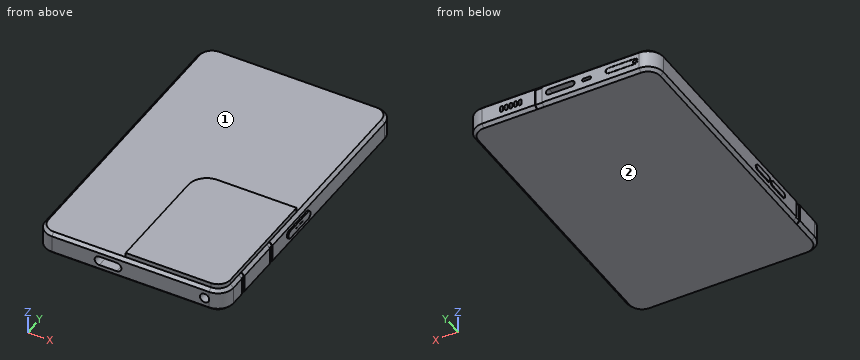
```python
from build123d import *

# Parameters (mm, degrees)
EXTRUDE_1_DEPTH        = 15
CHAMFER_7_SIZE         = 2
CHAMFER_8_SIZE         = 2
CUT_EXTRUDE_1_DEPTH    = 6
PATTERN_LINEAR_1_COUNT = 5
PATTERN_LINEAR_1_PITCH = 3
CUT_EXTRUDE_2_DEPTH    = 10
CUT_EXTRUDE_3_DEPTH    = 40
CUT_EXTRUDE_5_DEPTH    = 20
EXTRUDE_2_DEPTH        = 20
SKETCH_9_R             = 1.114563032
CUT_EXTRUDE_6_DEPTH    = 20
SKETCH_10_R            = 2.990185925
CUT_EXTRUDE_8_DEPTH    = 20
SKETCH_12_W            = 4.560479379
SKETCH_12_H            = 11
CUT_EXTRUDE_9_DEPTH    = 0.5
SKETCH_13_W            = 4.560479379
SKETCH_13_H            = 2.828427125
CUT_EXTRUDE_10_DEPTH   = 0.5
SKETCH_14_W            = 4.560479379
SKETCH_14_H            = 2.828427125
CUT_EXTRUDE_11_DEPTH   = 0.5
EXTRUDE_3_DEPTH        = 1
EXTRUDE_4_DEPTH        = 0.1
SKETCH_17_W            = 11
SKETCH_17_H            = 3
CUT_EXTRUDE_12_DEPTH   = 0.5
SKETCH_18_W            = 2.828427124
SKETCH_18_H            = 3
CUT_EXTRUDE_13_DEPTH   = 0.5
SKETCH_19_W            = 2.828427124
SKETCH_19_H            = 3
CUT_EXTRUDE_14_DEPTH   = 0.5
EXTRUDE_5_DEPTH        = 0.5
SKETCH_26_W            = 11
SKETCH_26_H            = 4
CUT_EXTRUDE_15_DEPTH   = 0.5
SKETCH_27_W            = 2.828427124
SKETCH_27_H            = 4
CUT_EXTRUDE_16_DEPTH   = 0.5
SKETCH_28_W            = 2.828427124
SKETCH_28_H            = 4
CUT_EXTRUDE_17_DEPTH   = 0.5
EXTRUDE_6_DEPTH        = 3


with BuildPart() as part:
    # 草图1 → 凸台-拉伸1 (new body)
    with BuildSketch(Plane.XY):
        with BuildLine():
            Line((-50.87521941, 95.847945747), (50.87521941, 95.847945747))
            ThreePointArc((50.87521941, 95.847945747), (57.946287222, 92.919013559), (60.87521941, 85.847945747))
            Line((60.87521941, 85.847945747), (60.87521941, -85.847945747))
            ThreePointArc((60.87521941, -85.847945747), (57.946287222, -92.919013559), (50.87521941, -95.847945747))
            Line((50.87521941, -95.847945747), (-50.87521941, -95.847945747))
            ThreePointArc((-50.87521941, -95.847945747), (-57.946287222, -92.919013559), (-60.87521941, -85.847945747))
            Line((-60.87521941, -85.847945747), (-60.87521941, 85.847945747))
            ThreePointArc((-60.87521941, 85.847945747), (-57.946287222, 92.919013559), (-50.87521941, 95.847945747))
        make_face()
    extrude(amount=EXTRUDE_1_DEPTH)

    # 倒角7
    chamfer_7_edges = [part.edges().sort_by_distance(p)[0] for p in [
        (0, 95.847945747, 0),
        (57.946287222, 92.919013559, 0),
        (60.87521941, 0, 0),
        (57.946287222, -92.919013559, 0),
        (0, -95.847945747, 0),
        (-57.946287222, -92.919013559, 0),
        (-60.87521941, 0, 0),
        (-57.946287222, 92.919013559, 0),
    ]]
    chamfer(chamfer_7_edges, length=CHAMFER_7_SIZE)

    # 倒角8
    chamfer_8_edges = [part.edges().sort_by_distance(p)[0] for p in [
        (57.946287222, 92.919013559, 15),
        (0, 95.847945747, 15),
        (-57.946287222, 92.919013559, 15),
        (-60.87521941, 0, 15),
        (-57.946287222, -92.919013559, 15),
        (0, -95.847945747, 15),
        (57.946287222, -92.919013559, 15),
        (60.87521941, 0, 15),
    ]]
    chamfer(chamfer_8_edges, length=CHAMFER_8_SIZE)

    # 草图4 → 切除-拉伸1 (cut)
    with BuildSketch(Plane(origin=(0, 95.847945747, 0), x_dir=(1, 0, 0), z_dir=(0, 1, 0))):
        with BuildLine():
            Line((25.184922723, -6.52592521), (25.184922723, -8.52592521))
            ThreePointArc((25.184922723, -8.52592521), (26.184922723, -9.52592521), (27.184922723, -8.52592521))
            Line((27.184922723, -8.52592521), (27.184922723, -6.52592521))
            ThreePointArc((27.184922723, -6.52592521), (26.184922723, -5.52592521), (25.184922723, -6.52592521))
        make_face()
    cut_extrude_1 = extrude(amount=-CUT_EXTRUDE_1_DEPTH, mode=Mode.SUBTRACT)

    # 阵列(线性)1: 切除-拉伸1 ×5
    with Locations(*[(i * PATTERN_LINEAR_1_PITCH, 0, 0) for i in range(1, PATTERN_LINEAR_1_COUNT)]):
        add(cut_extrude_1, mode=Mode.SUBTRACT)

    # 草图5 → 切除-拉伸2 (cut)
    with BuildSketch(Plane(origin=(0, 95.847945747, 0), x_dir=(1, 0, 0), z_dir=(0, 1, 0))):
        with BuildLine():
            Line((-18.674903906, -6.52592521), (-14.956626917, -6.52592521))
            ThreePointArc((-14.956626917, -6.52592521), (-13.956626917, -7.52592521), (-14.956626917, -8.52592521))
            Line((-14.956626917, -8.52592521), (-18.674903906, -8.52592521))
            ThreePointArc((-18.674903906, -8.52592521), (-19.674903906, -7.52592521), (-18.674903906, -6.52592521))
        make_face()
    extrude(amount=-CUT_EXTRUDE_2_DEPTH, mode=Mode.SUBTRACT)

    # 草图6 → 切除-拉伸3 (cut)
    with BuildSketch(Plane(origin=(0, 95.847945747, 0), x_dir=(1, 0, 0), z_dir=(0, 1, 0))):
        with BuildLine():
            Line((-7.094079035, -5.954899544), (7.600798966, -5.954899544))
            ThreePointArc((7.600798966, -5.954899544), (9.543225368, -7.897325947), (7.600798966, -9.839752349))
            Line((7.600798966, -9.839752349), (-7.094079035, -9.839752349))
            ThreePointArc((-7.094079035, -9.839752349), (-9.036505437, -7.897325947), (-7.094079035, -5.954899544))
        make_face()
    extrude(amount=-CUT_EXTRUDE_3_DEPTH, mode=Mode.SUBTRACT)

    # 草图7 → 切除-拉伸5 (cut)
    with BuildSketch(Plane(origin=(0, 95.847945747, 0), x_dir=(1, 0, 0), z_dir=(0, 1, 0))):
        with BuildLine():
            Line((-47.943352298, -5.954899544), (-31.050839612, -5.954899544))
            ThreePointArc((-31.050839612, -5.954899544), (-29.108413209, -7.897325947), (-31.050839612, -9.839752349))
            Line((-31.050839612, -9.839752349), (-47.943352298, -9.839752349))
            ThreePointArc((-47.943352298, -9.839752349), (-49.885778701, -7.897325947), (-47.943352298, -5.954899544))
        make_face()
    extrude(amount=-CUT_EXTRUDE_5_DEPTH, mode=Mode.SUBTRACT)

    # 草图8 → 凸台-拉伸2 (add)
    with BuildSketch(Plane(origin=(0, 75.847945747, 0), x_dir=(1, 0, 0), z_dir=(0, 1, 0))):
        with BuildLine():
            Line((-47.943352298, -6.108012441), (-31.050839612, -6.108012441))
            ThreePointArc((-31.050839612, -6.108012441), (-29.259969658, -7.898882395), (-31.050839612, -9.689752349))
            Line((-31.050839612, -9.689752349), (-47.943352298, -9.689752349))
            ThreePointArc((-47.943352298, -9.689752349), (-49.734222253, -7.898882395), (-47.943352298, -6.108012441))
        make_face()
    extrude(amount=EXTRUDE_2_DEPTH)

    # 草图9 → 切除-拉伸6 (cut)
    with BuildSketch(Plane(origin=(0, 95.847945747, 0), x_dir=(1, 0, 0), z_dir=(0, 1, 0))):
        with Locations(Location((-47.943352298, -7.898882395, 0), (0, 0, 270))):
            Circle(SKETCH_9_R)
    extrude(amount=-CUT_EXTRUDE_6_DEPTH, mode=Mode.SUBTRACT)

    # 草图10 → 切除-拉伸8 (cut)
    with BuildSketch(Plane.XZ.offset(95.847945747)):
        with Locations(Location((47.885033485, 7.5, 0), (0, 0, 270))):
            Circle(SKETCH_10_R)
        with BuildLine():
            Line((-8.945418448, 10.490185925), (-20.268797242, 10.490185925))
            ThreePointArc((-20.268797242, 10.490185925), (-23.258983167, 7.5), (-20.268797242, 4.509814075))
            Line((-20.268797242, 4.509814075), (-8.945418448, 4.509814075))
            ThreePointArc((-8.945418448, 4.509814075), (-5.955232523, 7.5), (-8.945418448, 10.490185925))
        make_face()
    extrude(amount=-CUT_EXTRUDE_8_DEPTH, mode=Mode.SUBTRACT)

    # 草图12 → 切除-拉伸9 (cut)
    with BuildSketch(Plane(origin=(0, 95.847945747, 0), x_dir=(1, 0, 0), z_dir=(0, 1, 0))):
        with Locations((14.272611391, -7.5)):
            Rectangle(SKETCH_12_W, SKETCH_12_H)
    extrude(amount=-CUT_EXTRUDE_9_DEPTH, mode=Mode.SUBTRACT)

    # 草图13 → 切除-拉伸10 (cut)
    with BuildSketch(Plane(origin=(0, 54.423972873, 54.423972873), x_dir=(1, 0, 0), z_dir=(0, 0.7071067811865452, 0.7071067811865498))):
        with Locations((14.272611391, 57.168130683)):
            Rectangle(SKETCH_13_W, SKETCH_13_H)
    extrude(amount=-CUT_EXTRUDE_10_DEPTH, mode=Mode.SUBTRACT)

    # 草图14 → 切除-拉伸11 (cut)
    with BuildSketch(Plane(origin=(0, 46.923972873, -46.923972873), x_dir=(1, 0, 0), z_dir=(0, 0.707106781186545, -0.70710678118655))):
        with Locations((14.272611391, -67.7747324)):
            Rectangle(SKETCH_14_W, SKETCH_14_H)
    extrude(amount=-CUT_EXTRUDE_11_DEPTH, mode=Mode.SUBTRACT)

    # 草图15 → 凸台-拉伸3 (add)
    with BuildSketch(Plane(origin=(60.87521941, 0, 0), x_dir=(0, 0, -1), z_dir=(1, 0, 0))):
        with BuildLine():
            Line((-10.846864794, -2.667254546), (-10.846864794, -22.628643405))
            ThreePointArc((-10.846864794, -22.628643405), (-8.265650718, -25.209857481), (-5.684436641, -22.628643405))
            Line((-5.684436641, -22.628643405), (-5.684436641, -2.667254546))
            ThreePointArc((-5.684436641, -2.667254546), (-8.265650718, -0.086040469), (-10.846864794, -2.667254546))
        make_face()
    extrude(amount=EXTRUDE_3_DEPTH)

    # 草图16 → 凸台-拉伸4 (add)
    with BuildSketch(Plane(origin=(61.87521941, 0, 0), x_dir=(0, 0, -1), z_dir=(1, 0, 0))):
        with BuildLine():
            Line((-8.465650718, -8.647948975), (-8.465650718, -16.647948975))
            ThreePointArc((-8.465650718, -16.647948975), (-8.265650718, -16.847948975), (-8.065650718, -16.647948975))
            Line((-8.065650718, -16.647948975), (-8.065650718, -8.647948975))
            ThreePointArc((-8.065650718, -8.647948975), (-8.265650718, -8.447948975), (-8.465650718, -8.647948975))
        make_face()
    extrude(amount=EXTRUDE_4_DEPTH)

    # 草图17 → 切除-拉伸12 (cut)
    with BuildSketch(Plane(origin=(60.87521941, 0, 0), x_dir=(0, 0, -1), z_dir=(1, 0, 0))):
        with Locations((-7.5, -74.859598899)):
            Rectangle(SKETCH_17_W, SKETCH_17_H)
        with Locations((-7.5, -43.013411788)):
            Rectangle(SKETCH_17_W, SKETCH_17_H)
    extrude(amount=-CUT_EXTRUDE_12_DEPTH, mode=Mode.SUBTRACT)

    # 草图18 → 切除-拉伸13 (cut)
    with BuildSketch(Plane(origin=(29.437609705, 0, -29.437609705), x_dir=(-0.7071067811865475, 0, -0.7071067811865477), z_dir=(0.7071067811865477, 0, -0.7071067811865475))):
        with Locations((-43.045280451, -43.013411788)):
            Rectangle(SKETCH_18_W, SKETCH_18_H)
        with Locations((-43.045280451, -74.859598899)):
            Rectangle(SKETCH_18_W, SKETCH_18_H)
    extrude(amount=-CUT_EXTRUDE_13_DEPTH, mode=Mode.SUBTRACT)

    # 草图19 → 切除-拉伸14 (cut)
    with BuildSketch(Plane(origin=(36.937609705, 0, 36.937609705), x_dir=(0.7071067811865498, 0, -0.7071067811865452), z_dir=(0.7071067811865452, 0, 0.7071067811865498))):
        with Locations((32.438678733, -43.013411788)):
            Rectangle(SKETCH_19_W, SKETCH_19_H)
        with Locations((32.438678733, -74.859598899)):
            Rectangle(SKETCH_19_W, SKETCH_19_H)
    extrude(amount=-CUT_EXTRUDE_14_DEPTH, mode=Mode.SUBTRACT)

    # 草图25 → 凸台-拉伸5 (add)
    with BuildSketch(Plane.ZY.offset(60.87521941)):
        with BuildLine():
            Line((5.092196702, -20.703608048), (5.092196702, -32.703608048))
            ThreePointArc((5.092196702, -32.703608048), (6.87745097, -34.488862317), (8.662705239, -32.703608048))
            Line((8.662705239, -32.703608048), (8.662705239, -20.703608048))
            ThreePointArc((8.662705239, -20.703608048), (6.87745097, -18.91835378), (5.092196702, -20.703608048))
        make_face()
        with BuildLine():
            Line((5.092196702, -37.703608048), (5.092196702, -49.703608048))
            ThreePointArc((5.092196702, -49.703608048), (6.87745097, -51.488862317), (8.662705239, -49.703608048))
            Line((8.662705239, -49.703608048), (8.662705239, -37.703608048))
            ThreePointArc((8.662705239, -37.703608048), (6.87745097, -35.91835378), (5.092196702, -37.703608048))
        make_face()
    extrude(amount=EXTRUDE_5_DEPTH)

    # 草图26 → 切除-拉伸15 (cut)
    with BuildSketch(Plane.ZY.offset(60.87521941)):
        with Locations((7.5, -67.142133824)):
            Rectangle(SKETCH_26_W, SKETCH_26_H)
    extrude(amount=-CUT_EXTRUDE_15_DEPTH, mode=Mode.SUBTRACT)

    # 草图27 → 切除-拉伸16 (cut)
    with BuildSketch(Plane(origin=(-36.937609705, 0, 36.937609705), x_dir=(0.7071067811865498, 0, 0.7071067811865452), z_dir=(-0.7071067811865452, 0, 0.7071067811865498))):
        with Locations((-32.438678733, -67.142133824)):
            Rectangle(SKETCH_27_W, SKETCH_27_H)
    extrude(amount=-CUT_EXTRUDE_16_DEPTH, mode=Mode.SUBTRACT)

    # 草图28 → 切除-拉伸17 (cut)
    with BuildSketch(Plane(origin=(-29.437609705, 0, -29.437609705), x_dir=(-0.7071067811865475, 0, 0.7071067811865477), z_dir=(-0.7071067811865477, 0, -0.7071067811865475))):
        with Locations((43.045280451, -67.142133824)):
            Rectangle(SKETCH_28_W, SKETCH_28_H)
    extrude(amount=-CUT_EXTRUDE_17_DEPTH, mode=Mode.SUBTRACT)

    # 草图30 → 凸台-拉伸6 (add)
    with BuildSketch(Plane.XY.offset(15)):
        with BuildLine():
            Line((-4.346185338, -93.847945747), (-4.346185338, -22.755058652))
            ThreePointArc((-4.346185338, -22.755058652), (-0.831466712, -14.269777278), (7.653814662, -10.755058652))
            Line((7.653814662, -10.755058652), (58.87521941, -10.755058652))
            Line((58.87521941, -10.755058652), (58.87521941, -85.847945747))
            ThreePointArc((58.87521941, -85.847945747), (56.532073659, -91.504799996), (50.87521941, -93.847945747))
            Line((50.87521941, -93.847945747), (-4.346185338, -93.847945747))
        make_face()
    extrude(amount=EXTRUDE_6_DEPTH)


solid = part.part
```
The model under review builds one solid part; all positions refer to its coordinate system, in mm. Face numbers are marked on the shaded views. A direction names the side the tool comes from. Coordinates: 2 decimals unless noted, no trailing zeros. Loops run counter-clockwise (first coordinate to the right, second up) from the corner with the lowest first, then second, coordinate; pieces in that order, holes last. Notation, with made-up numbers: (76, 19.5) -> (117, 19.5) arc R20 cw to (117, 31.5) -> close; hole circle Ø1 at (-16, -18). An arc over 180 degrees is marked (long way). Answer as CSV lines item,"result".
Item 1: Insertion check: pin 1 (1 mm diameter, centred on y = 92, z = 7, fed in from +X); pin 2 (0.7 mm diameter, centred on x = -59.5, z = 10.5, fed in from +Y); pin 3 (1 mm diameter, centred on y = 92.5, z = 7.5, fed in from +X). Each pin has a flat end and moves straight along its axis. Give the tip position at first contact, or say it passes through.
Results below:
pin 1,"stops at x = 59.12"
pin 2,"stops at y = 91.46"
pin 3,"stops at x = 58.76"
Item 2: Take a section at A-A, the plane x = 19. State the section outline as (y, z) points, and give its area (3 significant figures).
Results below:
outline,"(-95.85, 2) -> (-93.85, 0) -> (93.85, 0) -> (95.85, 2) -> (95.85, 13) -> (93.85, 15) -> (-10.76, 15) -> (-10.76, 18) -> (-93.85, 18) -> (-93.85, 15) -> (-95.85, 13) -> close"
area,"3,120 mm2"
Item 3: For L1, parallel to X at y = -81.5, z = 7.5; L2, parallel to Y at x = -5, z = 6.5; L3, parallel to Y at x = -7, z = 8.75, list the stretches that pass through material, from the lowest coordinate up.
Results below:
L1,"x = -60.88 to -23.26, -5.96 to 44.89, 50.88 to 60.88"
L2,"y = -95.85 to 55.85"
L3,"y = -75.85 to 55.85"
Item 4: Take a section at B-B, the plane x = 4. State the section outline as (y, z) points.
Results below:
outline,"(-95.85, 2) -> (-93.85, 0) -> (93.85, 0) -> (95.85, 2) -> (95.85, 5.95) -> (55.85, 5.95) -> (55.85, 9.84) -> (95.85, 9.84) -> (95.85, 13) -> (93.85, 15) -> (-11.32, 15) -> (-11.32, 18) -> (-93.85, 18) -> (-93.85, 15) -> (-95.85, 13) -> close"
Item 5: Machinability: for the marked faces 1 and 2, which of the approach directions +Z, -Z, +X, -X, +Y, -Y give a long, thin tool a straight path to every point of the face, cutting with its end or side? Answer none if there is none.
Results below:
face 1,"+Z, -X, +Y"
face 2,"-Z, +X, -X, +Y, -Y"
